Geometry check sheet. Reference: the model listing, model coordinates, mm. Face numbers are marked on the shaded views. A direction names the side the tool comes from. Round coordinates to 2 decimals unless told otherwise and drop trailing zeros. Order: outer loops, then holes, each group sorted by start corner. A loop starts at its lowest first (then second) coordinate and runs counter-clockwise, first axis right, second up.
(1) Cross-section at B-B on x = 7. Enter the section's corners in (y, z).
(2) Set-up check for the marked faces 1 and 2: record each of +Z, -Z, +X, -X, +Y, -Y from which the full face is reachable in a straight line by a thin tool's end or side.
(3) Gauge pin test, flat ends, axial feed: P1, Ø8.5, axis at y = 76.2, z = -58.74, coming from the +X side; P2, Ø1, axis at x = -24.5, y = 755.5, coming from the -Z side; P3, Ø24, axis at x = -9, y = 496, coming from the -Z side. Record the tip position at first contact, or that the pin passes through.
(4) Thickness scan on L1, parallel to X at y = 830, z = -14.5 (1 decimal); L2, parallel to Z at x = -32.1, y = 355.6; L3, parallel to Z at x = 5, y = 314.5. Record the ranges inside material, lowest first.
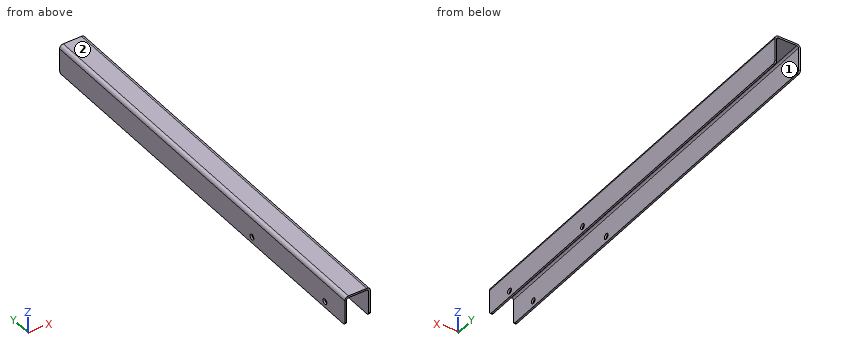
from build123d import *

# Parameters (mm, degrees)
SKETCH1_W                      = 57.15
SKETCH1_H                      = 1092.2
BASE_FLANGE1_DEPTH             = 4.7625
EDGE_FLANGE1_STRIP_W           = 28.575
EDGE_FLANGE1_STRIP_H           = 4.7625
EDGE_FLANGE1_STRIP_CUT_DEPTH   = 1092.2
EDGE_FLANGE1_STRIP_2_W         = 28.575
EDGE_FLANGE1_STRIP_2_H         = 4.7625
EDGE_FLANGE1_STRIP_CUT_2_DEPTH = 1092.2
EDGE_FLANGE1_DEPTH             = 1092.2
EDGE_FLANGE1_BEND_DEPTH        = 1092.2
F_1_2_CLEARANCE_HOLE1_D        = 14.2875
FILLET1_R                      = 6.35


# Sheet-metal steps are written as plain solids
with BuildPart() as part:
    # Sketch1 → Base-Flange1 (new body)
    with BuildSketch(Plane.XY):
        with Locations((0, 546.1)):
            Rectangle(SKETCH1_W, SKETCH1_H)
    extrude(amount=-BASE_FLANGE1_DEPTH)

    # Edge-Flange1 strip (across the edge) → Edge-Flange1 strip cut (cut)
    with BuildSketch(Plane(origin=(-28.575, 0, -4.7625), x_dir=(1, 0, 0), z_dir=(0, 1, 0))):
        with Locations((-9.525, -2.38125)):
            Rectangle(EDGE_FLANGE1_STRIP_W, EDGE_FLANGE1_STRIP_H)
    extrude(amount=EDGE_FLANGE1_STRIP_CUT_DEPTH, mode=Mode.SUBTRACT)

    # Edge-Flange1 strip 2 (across the edge) → Edge-Flange1 strip cut 2 (cut)
    with BuildSketch(Plane(origin=(28.575, 1092.2, -4.7625), x_dir=(-1, 0, 0), z_dir=(0, -1, 0))):
        with Locations((-9.525, -2.38125)):
            Rectangle(EDGE_FLANGE1_STRIP_2_W, EDGE_FLANGE1_STRIP_2_H)
    extrude(amount=EDGE_FLANGE1_STRIP_CUT_2_DEPTH, mode=Mode.SUBTRACT)

    # Edge-Flange1 section (across the edge) → Edge-Flange1 (add)
    with BuildSketch(Plane(origin=(-28.575, 0, -4.7625), x_dir=(1, 0, 0), z_dir=(0, 1, 0))):
        with BuildLine():
            Line((-4.7625, 4.7625), (-4.7625, 69.85))
            Line((-4.7625, 69.85), (0, 69.85))
            Line((0, 69.85), (0, 4.7625))
            ThreePointArc((0, 4.7625), (1.394903955, 1.394903955), (4.7625, 0))
            Line((4.7625, 0), (4.7625, -4.7625))
            ThreePointArc((4.7625, -4.7625), (-1.972692091, -1.972692091), (-4.7625, 4.7625))
        make_face()
    extrude(amount=EDGE_FLANGE1_DEPTH)

    # Edge-Flange1 section 2 (across the edge) → Edge-Flange1 bend (add)
    with BuildSketch(Plane(origin=(28.575, 1092.2, -4.7625), x_dir=(-1, 0, 0), z_dir=(0, -1, 0))):
        with BuildLine():
            Line((-4.7625, 4.7625), (-4.7625, 69.85))
            Line((-4.7625, 69.85), (0, 69.85))
            Line((0, 69.85), (0, 4.7625))
            ThreePointArc((0, 4.7625), (1.394903955, 1.394903955), (4.7625, 0))
            Line((4.7625, 0), (4.7625, -4.7625))
            ThreePointArc((4.7625, -4.7625), (-1.972692091, -1.972692091), (-4.7625, 4.7625))
        make_face()
    extrude(amount=EDGE_FLANGE1_BEND_DEPTH)

    # 1/2 Clearance Hole1 (through all)
    with Locations(Plane(origin=(33.3375, 0, 0), x_dir=(0, 0, -1), z_dir=(1, 0, 0))):
        with Locations((58.7375, 76.2), (58.7375, 355.6)):
            Hole(F_1_2_CLEARANCE_HOLE1_D / 2)

    # Fillet1
    fillet1_edges = [part.edges().sort_by_distance(p)[0] for p in [
        (-30.95625, 0, -74.6125),
        (-30.95625, 1092.2, -74.6125),
        (30.95625, 1092.2, -74.6125),
        (30.95625, 0, -74.6125),
    ]]
    fillet(fillet1_edges, radius=FILLET1_R)


solid = part.part
Found:
1. outline: (0, -4.76) - (1092.2, -4.76) - (1092.2, 0) - (0, 0) - close
2. face 1: -Z, +Y, -Y
2. face 2: +Z, +X, -X, +Y, -Y
3. P1: passes through
3. P2: stops at z = -4.91
3. P3: stops at z = -4.76
4. L1: x = -33.3 to -28.6, 28.6 to 33.3
4. L2: z = -74.61 to -65.88, -51.59 to -4.83
4. L3: z = -4.76 to 0
